Here's how the part is built. I have some questions about the finished solid (model axes, mm). Round coordinates to 2 decimals unless told otherwise and drop trailing zeros. Order: outer loops, then holes, each group sorted by start corner. A loop starts at its lowest first (then second) coordinate and runs counter-clockwise, first axis right, second up. Notation, with made-up numbers: M 35,-15.5 L 54,-15.5 A29 cw 54,18.5 Z; hole C 78.25,42.25 d3. An arc over 180 degrees is marked long. Write item = value, one per line. Start each with the question number.
Item 1: We'd pull the mould along Y, two halves only. Please class faces 1 (the face through (2, 61, 3.124)), 2 (the face through (3.969, 7, 4)): pulls with the +Y half, pulls with the -Y half, needs draft (parallel to the pull), parting line crosses it, or undercut.
Item 2: Please list where these lines run through material, in increasing order: L1, parallel to X at y = 47, z = -2.75; L2, parallel to Z at x = 21, y = 24.5; L3, parallel to Y at x = 28, z = -12.25.
Item 3: I'm going to push flat-ended pins straight in: P1, Ø0.8, axis at x = 3, y = 2.5, coming from the +Z side; P2, Ø1.7, axis at x = 29.5, z = 2, coming from the -Y side; P3, Ø1.7, axis at x = 29, y = 45.5, coming from the -Z side; P4, Ø1.5, axis at x = 25.5, z = -1, coming from the -Y side. Where does each tip first touch, or does it pass through?
Item 4: I want a section at C-C, the plane y = 53. List the corners of the cut face in (x, z) for me, plus the area to 3 significant figures.
Item 5: I want a section at A-A, the plane z = -2.5. List the corners of the cut face in (x, y) for me.
Item 6: I want a section at D-D, the plane x = 3. State how many separate pieces and enclosed holes the cut face has, plus the area to 3 significant figures.
```python
from build123d import *

# Parameters (mm, degrees)
F1_DEPTH = 7.9375
F2_R     = 3.96874
F3_W     = 3.96875
F3_H     = 23.8125
F4_DEPTH = 15.875
F5_W     = 1.56845
F5_H     = 1.6891
F5_W_2   = 1.6891
F5_H_2   = 1.56845
F6_DEPTH = 31.75


# Not quite as in the source:
# - a fillet or chamfer is up to 0.001 mm smaller than in the source, because OpenCascade refuses the exact size


with BuildPart() as f1:
    # F0 (on Top) → F1 (new body)
    with BuildSketch(Plane.XY):
        Polygon((0, 63.5), (0, 0), (3.96875, 0), (3.96875, 9.525), (27.78125, 9.525), (27.78125, 0), (31.75, 0), (31.75, 63.5), (27.78125, 63.5), (27.78125, 39.6875), (3.96875, 39.6875), (3.96875, 63.5), align=None)
    extrude(amount=F1_DEPTH)

    # F2 (radius 3.96875 in the source; OpenCascade refuses exactly that, so slightly less here)
    f2_edges = [f1.edges().sort_by_distance(p)[0] for p in [
        (15.875, 39.6875, 7.9375),
        (15.875, 39.6875, 0),
        (1.984375, 63.5, 7.9375),
        (29.765625, 63.5, 7.9375),
        (1.984375, 0, 7.9375),
        (1.984375, 0, 0),
        (29.765625, 0, 7.9375),
        (29.765625, 0, 0),
        (15.875, 9.525, 7.9375),
        (15.875, 9.525, 0),
    ]]
    fillet(f2_edges, radius=F2_R)

    # F3 (on face) → F4 (join)
    with BuildSketch(Plane(origin=(0, 0, 0), x_dir=(1, 0, 0), z_dir=(0, 0, -1))):
        with Locations((29.765625, -51.59375)):
            Rectangle(F3_W, F3_H)
        with Locations((1.984375, -51.59375)):
            Rectangle(F3_W, F3_H)
    extrude(amount=F4_DEPTH)

    # F5 (on face) → F6 (cut, through all)
    with BuildSketch(Plane(origin=(0, 0, 0), x_dir=(0, -1, 0), z_dir=(-1, 0, 0))):
        with Locations((-5.597525, 3.96875)):
            Rectangle(F5_W, F5_H)
        with Locations((-3.96875, 3.96875)):
            Rectangle(F5_W_2, F5_H)
        with Locations((-3.96875, 2.339975)):
            Rectangle(F5_W_2, F5_H_2)
        with Locations((-2.339975, 3.96875)):
            Rectangle(F5_W, F5_H)
        with Locations((-3.96875, 5.597525)):
            Rectangle(F5_W_2, F5_H_2)
        with BuildLine():
            Line((-63.5, -15.875), (-59.53125, -15.875))
            ThreePointArc((-59.53125, -15.875), (-62.3375800378, -14.7125800378), (-63.5, -11.90625))
            Line((-63.5, -11.90625), (-63.5, -15.875))
        make_face()
        with BuildLine():
            Line((-59.53125, -15.875), (-39.6875, -15.875))
            Line((-39.6875, -15.875), (-39.6875, 0))
            Line((-39.6875, 0), (-56.935957382, -14.9088210299))
            ThreePointArc((-56.935957382, -14.9088210299), (-58.146597916, -15.6256202651), (-59.53125, -15.875))
        make_face()
        with Locations((-57.902475, -11.90625)):
            Rectangle(F5_W, F5_H)
        with Locations((-59.53125, -11.90625)):
            Rectangle(F5_W_2, F5_H)
        with Locations((-59.53125, -10.277475)):
            Rectangle(F5_W_2, F5_H_2)
        with Locations((-61.160025, -11.90625)):
            Rectangle(F5_W, F5_H)
        with Locations((-59.53125, -13.535025)):
            Rectangle(F5_W_2, F5_H_2)
        with Locations((-59.53125, 5.597525)):
            Rectangle(F5_W_2, F5_H_2)
        with Locations((-59.53125, 3.96875)):
            Rectangle(F5_W_2, F5_H)
        with Locations((-61.160025, 3.96875)):
            Rectangle(F5_W, F5_H)
        with Locations((-57.902475, 3.96875)):
            Rectangle(F5_W, F5_H)
        with Locations((-59.53125, 2.339975)):
            Rectangle(F5_W_2, F5_H_2)
        with Locations((-43.65625, 5.597525)):
            Rectangle(F5_W_2, F5_H_2)
        with Locations((-43.65625, 3.96875)):
            Rectangle(F5_W_2, F5_H)
        with Locations((-45.285025, 3.96875)):
            Rectangle(F5_W, F5_H)
        with Locations((-42.027475, 3.96875)):
            Rectangle(F5_W, F5_H)
        with Locations((-43.65625, 2.339975)):
            Rectangle(F5_W_2, F5_H_2)
    extrude(amount=-F6_DEPTH, mode=Mode.SUBTRACT)


solid = f1.part
```
Filled in:
q1.face_1 = undercut
q1.face_2 = needs draft
q2.L1 = 0 to 3.97, 27.78 to 31.75
q2.L2 = 0 to 7.94
q2.L3 = 53.86 to 57.12, 61.94 to 63.49
q3.P1 = 7.79
q3.P2 = 0.16
q3.P3 = -5.76
q3.P4 = through
q4.outline = M 0,-11.51 L 3.97,-11.51 L 3.97,7.94 L 0,7.94 Z; M 27.78,-11.51 L 31.75,-11.51 L 31.75,7.94 L 27.78,7.94 Z
q4.area = 154 mm^2
q5.outline = M 0,42.58 L 3.97,42.58 L 3.97,63.5 L 0,63.5 Z; M 27.78,42.58 L 31.75,42.58 L 31.75,63.5 L 27.78,63.5 Z
q6.separate_pieces = 1
q6.enclosed_holes = 4
q6.area = 669 mm^2
